Geometry: final body of the model. Coordinates: model frame, mm. Face numbers are marked on the shaded views. A direction names the side the tool comes from. Give positions to 0.01 mm unless a question says otherwise; leave off trailing zeros. Write each loop counter-clockwise with the first axis right and the second up, starting at its lowest first coordinate (ties: lowest second). Pieces come first, ordered by that corner, then holes. Notation, with made-up numbers: (3.5, -28) -> (58.5, -28) arc R32 cw to (58.5, -1) -> close; hole circle Ø7 at (-23.5, 13). An arc over 180 degrees is marked (long way). Answer in a Markdown table with one row per item. Add a question column.
Item 1: Section query A-A on x = 0. Output: boundary loops of the cut face in (y, z).
Item 2: Material intervals for probe 1 along Y at (x, z) = (0, 3.75); probe 2 along Y at (x, z) = (28, 9.5); probe 3 along Z at (x, y) = (-45, -20.5), sorted ascending. Write a range as from..to.
Item 3: First-contact query: P1, Ø4, axis at x = 39, y = 6, coming from the +Z side; P2, Ø3, axis at y = 8, z = 56.5, coming from the -X side; P3, Ø12, axis at x = 11, z = 77.5, coming from the +Y side. Flat tips, straight axial feed; report the tip coordinate or a pass-through.
Item 4: Section query B-B on z = 11.5. Output: boundary loops of the cut face in (x, y).
Item 5: Section query D-D on y = 0. Output: boundary loops of the cut face in (x, z).
Item 6: Access query for the marked faces 1 and 2. Directions: +Z, -Z, +X, -X, +Y, -Y. A direction counts if a zero-diameter tool reaches every point of the face in a straight line with its end or side. Return the directions, or none.
Item 7: Section query C-C on y = -17.5. Output: boundary loops of the cut face in (x, z), plus the area to 3 significant figures.
```python
from build123d import *

# Parameters (mm, degrees)
F0_R     = 50
F0_R_2   = 6
F1_DEPTH = 15
F2_R     = 25
F3_DEPTH = 75


with BuildPart() as f1:
    # F0 (on Top) → F1 (new body)
    with BuildSketch(Plane.XY):
        Circle(F0_R)
        with Locations((-30.310889, -17.5)):
            Circle(F0_R_2, mode=Mode.SUBTRACT)
        with Locations((0, -35)):
            Circle(F0_R_2, mode=Mode.SUBTRACT)
        with Locations((30.310889, -17.5)):
            Circle(F0_R_2, mode=Mode.SUBTRACT)
        with Locations((-30.310889, 17.5)):
            Circle(F0_R_2, mode=Mode.SUBTRACT)
        with Locations((30.310889, 17.5)):
            Circle(F0_R_2, mode=Mode.SUBTRACT)
        with Locations((0, 35)):
            Circle(F0_R_2, mode=Mode.SUBTRACT)
    extrude(amount=F1_DEPTH)

    # F2 (on face) → F3 (join)
    with BuildSketch(Plane.XY.offset(15)):
        Circle(F2_R)
    extrude(amount=F3_DEPTH)


solid = f1.part
```
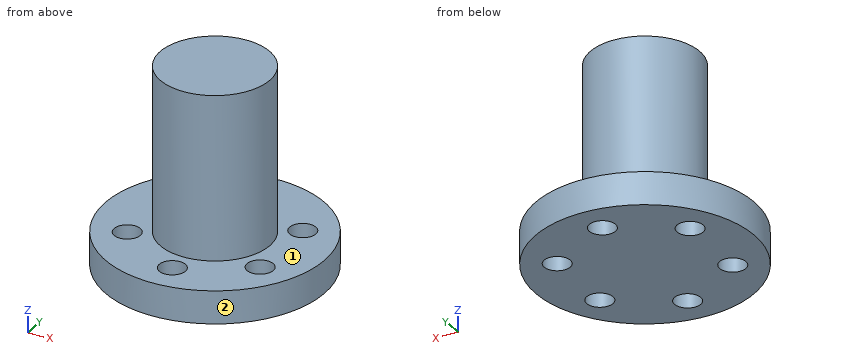
Findings below:
| question | item | result |
|---|---|---|
| 1 | outline | (-50, 0) -> (-41, 0) -> (-41, 15) -> (-50, 15) -> close; (-29, 0) -> (29, 0) -> (29, 15) -> (25, 15) -> (25, 90) -> (-25, 90) -> (-25, 15) -> (-29, 15) -> close; (41, 0) -> (50, 0) -> (50, 15) -> (41, 15) -> close |
| 2 | probe 1 | y = -50..-41, -29..29, 41..50 |
| 2 | probe 2 | y = -41.42..-23.04, -11.96..11.96, 23.04..41.42 |
| 2 | probe 3 | z = 0..15 |
| 3 | P1 | stops at z = 15 |
| 3 | P2 | stops at x = -24.14 |
| 3 | P3 | stops at y = 24.49 |
| 4 | outline | circle Ø100 at (0, 0); hole circle Ø12 at (-30.31, -17.5); hole circle Ø12 at (-30.31, 17.5); hole circle Ø12 at (0, -35); hole circle Ø12 at (0, 35); hole circle Ø12 at (30.31, -17.5); hole circle Ø12 at (30.31, 17.5) |
| 5 | outline | (-50, 0) -> (50, 0) -> (50, 15) -> (25, 15) -> (25, 90) -> (-25, 90) -> (-25, 15) -> (-50, 15) -> close |
| 6 | face 1 | +Z |
| 6 | face 2 | +Z, -Z |
| 7 | outline | (-46.84, 0) -> (-36.31, 0) -> (-36.31, 15) -> (-46.84, 15) -> close; (-24.31, 0) -> (24.31, 0) -> (24.31, 15) -> (17.85, 15) -> (17.85, 90) -> (-17.85, 90) -> (-17.85, 15) -> (-24.31, 15) -> close; (36.31, 0) -> (46.84, 0) -> (46.84, 15) -> (36.31, 15) -> close |
| 7 | area | 3,720 mm^2 |
